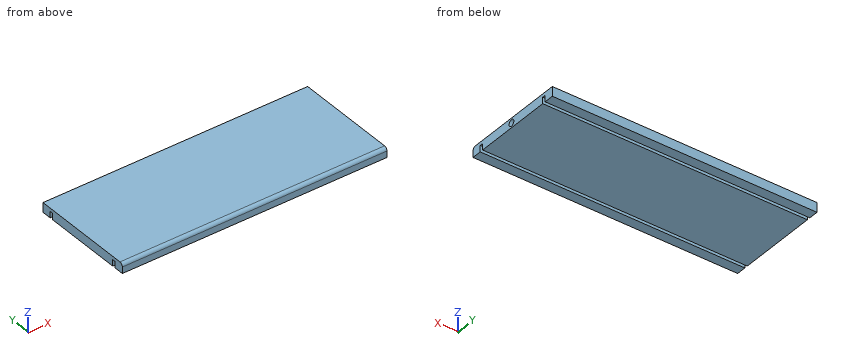
from build123d import *

# Parameters (mm, degrees)
F0_W     = 83
F0_H     = 33
F1_DEPTH = 3
F2_W     = 1
F2_H     = 2
F3_DEPTH = 83.001
F4_W     = 2.98905
F4_H     = 25
F5_DEPTH = 2
F6_R     = 1
F7_DEPTH = 25
F8_R     = 1


with BuildPart() as f1:
    # F0 (on Top) → F1 (new body)
    with BuildSketch(Plane.XY):
        with Locations((-19.543798, -15.713293)):
            Rectangle(F0_W, F0_H)
    extrude(amount=F1_DEPTH)

    # F2 (on face) → F3 (cut, through all)
    with BuildSketch(Plane.YZ.offset(21.956202)):
        with Locations((-28.713293, 1)):
            Rectangle(F2_W, F2_H)
        with Locations((-2.713293, 1)):
            Rectangle(F2_W, F2_H)
    extrude(amount=-F3_DEPTH, mode=Mode.SUBTRACT)

    # F4 (on face) → F5 (join)
    with BuildSketch(Plane(origin=(0, 0, 0), x_dir=(1, 0, 0), z_dir=(0, 0, -1))):
        with Locations((-45.065695, 15.713293)):
            Rectangle(F4_W, F4_H)
    extrude(amount=-F5_DEPTH)

    # F6 (on face) → F7 (cut)
    with BuildSketch(Plane.YZ.offset(21.956202)):
        with Locations((-16.213293, 1.5)):
            Circle(F6_R)
    extrude(amount=-F7_DEPTH, mode=Mode.SUBTRACT)

    # F8
    f8_edges = [f1.edges().sort_by_distance(p)[0] for p in [
        (-19.543798, -32.213293, 3),
    ]]
    fillet(f8_edges, radius=F8_R)


solid = f1.part
Geometry: final body of the model. Coordinates: model frame, mm. Coordinates: 2 decimals unless noted, no trailing zeros. Order: outer loops, then holes, each group sorted by start corner. A loop starts at its lowest first (then second) coordinate and runs counter-clockwise, first axis right, second up.
(1) Section query B-B (x = 13). Return the cut outline in (y, z).
(2) Section query C-C (x = -36.5). Return the cut outline in (y, z), plus the area to 3 significant figures.
(3) Material intervals for probe 1 along Y at (x, z) = (-22.5, 0.75); probe 2 along Z at (x, y) = (0.5, -3); probe 3 along Y at (x, z) = (3.5, 1.9), sorted ascending.
(4) Section query A-A (z = 1.5). Return the cut outline in (x, y).
Solution:
1. outline: (-32.21, 0) - (-29.21, 0) - (-29.21, 2) - (-28.21, 2) - (-28.21, 0) - (-3.21, 0) - (-3.21, 2) - (-2.21, 2) - (-2.21, 0) - (0.79, 0) - (0.79, 3) - (-31.21, 3) arc R1 ccw to (-32.21, 2) - close; hole circle Ø2 at (-16.21, 1.5)
2. outline: (-32.21, 0) - (-29.21, 0) - (-29.21, 2) - (-28.21, 2) - (-28.21, 0) - (-3.21, 0) - (-3.21, 2) - (-2.21, 2) - (-2.21, 0) - (0.79, 0) - (0.79, 3) - (-31.21, 3) arc R1 ccw to (-32.21, 2) - close
2. area: 94.8 mm2
3. probe 1: y = -32.21 to -29.21, -28.21 to -3.21, -2.21 to 0.79
3. probe 2: z = 2 to 3
3. probe 3: y = -32.21 to -29.21, -28.21 to -17.13, -15.3 to -3.21, -2.21 to 0.79
4. outline: (-61.04, -32.21) - (21.96, -32.21) - (21.96, -29.21) - (-61.04, -29.21) - close; (-61.04, -28.21) - (21.96, -28.21) - (21.96, -17.21) - (-3.04, -17.21) - (-3.04, -15.21) - (21.96, -15.21) - (21.96, -3.21) - (-61.04, -3.21) - close; (-61.04, -2.21) - (21.96, -2.21) - (21.96, 0.79) - (-61.04, 0.79) - close
